from build123d import *

# Parameters (mm, degrees)
BOSS_EXTRUDE1_DEPTH     = 28
CUT_EXTRUDE1_DEPTH      = 19
CUT_EXTRUDE1_DEPTH_BACK = 52
SKETCH3_R               = 2.75
BOSS_EXTRUDE2_DEPTH     = 2
SKETCH5_R               = 2.25
CUT_EXTRUDE2_DEPTH      = 50
CUT_EXTRUDE3_DEPTH      = 2
MIRROR3_COPY_1_DEPTH    = 2
SKETCH7_R               = 7.5
CUT_EXTRUDE4_DEPTH      = 10
BOSS_EXTRUDE3_DEPTH     = 4
CHAMFER1_SIZE           = 4
SKETCH9_R               = 3.3
SKETCH9_R_2             = 2.75
BOSS_EXTRUDE4_DEPTH     = 1.5
CHAMFER2_SIZE           = 1.5
CHAMFER3_SIZE           = 1.5
SKETCH10_W              = 16
SKETCH10_H              = 4
BOSS_EXTRUDE5_DEPTH     = 28


with BuildPart() as part:
    # Sketch2 → Boss-Extrude1 (new body)
    with BuildSketch(Plane.XY):
        with BuildLine():
            ThreePointArc((-59.5, 14), (-56.717514421, 20.717514421), (-50, 23.5))
            Line((-50, 23.5), (-36, 23.5))
            Line((-36, 23.5), (-36, -19.5))
            Line((-36, -19.5), (-24, -19.5))
            Line((-24, -19.5), (-24, 23.5))
            Line((-24, 23.5), (50, 23.5))
            ThreePointArc((50, 23.5), (56.717514421, 20.717514421), (59.5, 14))
            Line((59.5, 14), (59.5, -14))
            ThreePointArc((59.5, -14), (56.717514421, -20.717514421), (50, -23.5))
            Line((50, -23.5), (-50, -23.5))
            ThreePointArc((-50, -23.5), (-56.717514421, -20.717514421), (-59.5, -14))
            Line((-59.5, -14), (-59.5, 14))
        make_face()
        with BuildLine():
            ThreePointArc((50, -19.5), (53.889087297, -17.889087297), (55.5, -14))
            Line((55.5, -14), (55.5, 14))
            ThreePointArc((55.5, 14), (53.889087297, 17.889087297), (50, 19.5))
            Line((50, 19.5), (-20, 19.5))
            Line((-20, 19.5), (-20, -19.5))
            Line((-20, -19.5), (50, -19.5))
        make_face(mode=Mode.SUBTRACT)
        with BuildLine():
            Line((-55.5, -14), (-55.5, 14))
            ThreePointArc((-55.5, 14), (-53.889087297, 17.889087297), (-50, 19.5))
            Line((-50, 19.5), (-40, 19.5))
            Line((-40, 19.5), (-40, -19.5))
            Line((-40, -19.5), (-50, -19.5))
            ThreePointArc((-50, -19.5), (-53.889087297, -17.889087297), (-55.5, -14))
        make_face(mode=Mode.SUBTRACT)
    extrude(amount=BOSS_EXTRUDE1_DEPTH)

    # Sketch3 → Cut-Extrude1 (cut, two sides: drawn at the far end of the back side and taken through both)
    with BuildSketch(Plane(origin=(-36, 0, 0), x_dir=(0, 0, -1), z_dir=(1, 0, 0)).offset(-CUT_EXTRUDE1_DEPTH_BACK)):
        with Locations(Location((-14, 1.5, 0), (0, 0, 180))):
            Circle(SKETCH3_R)
    extrude(amount=CUT_EXTRUDE1_DEPTH + CUT_EXTRUDE1_DEPTH_BACK, mode=Mode.SUBTRACT)

    # Sketch4 → Boss-Extrude2 (add)
    with BuildSketch(Plane.XY.offset(28)):
        with BuildLine():
            Line((50, 23.5), (-36, 23.5))
            Line((-36, 23.5), (-50, 23.5))
            ThreePointArc((-50, 23.5), (-56.717514421, 20.717514421), (-59.5, 14))
            Line((-59.5, 14), (-59.5, -14))
            ThreePointArc((-59.5, -14), (-56.717514421, -20.717514421), (-50, -23.5))
            Line((-50, -23.5), (50, -23.5))
            ThreePointArc((50, -23.5), (56.717514421, -20.717514421), (59.5, -14))
            Line((59.5, -14), (59.5, 14))
            ThreePointArc((59.5, 14), (56.717514421, 20.717514421), (50, 23.5))
        make_face()
    extrude(amount=BOSS_EXTRUDE2_DEPTH)

    # Sketch5 → Cut-Extrude2 (cut)
    with BuildSketch(Plane(origin=(0, 23.5, 0), x_dir=(1, 0, 0), z_dir=(0, 1, 0))):
        with Locations(Location((-50, -15, 0), (0, 0, 270))):
            Circle(SKETCH5_R)
    cut_extrude2 = extrude(amount=-CUT_EXTRUDE2_DEPTH, mode=Mode.SUBTRACT)

    # Sketch6 → Cut-Extrude3 (cut, symmetric)
    with BuildSketch(Plane(origin=(0, -19.5, 0), x_dir=(1, 0, 0), z_dir=(0, 1, 0))):
        Polygon((-50, -19.272391992), (-46.3, -17.136195996), (-46.3, -12.863804004), (-50, -10.727608008), (-53.7, -12.863804004), (-53.7, -17.136195996), align=None)
    cut_extrude3 = extrude(amount=CUT_EXTRUDE3_DEPTH, both=True, mode=Mode.SUBTRACT)

    # Mirror1: Cut-Extrude2 across plane
    add(cut_extrude2.mirror(Plane(origin=(0, 0, 0), x_dir=(0, 0, 1), z_dir=(1, 0, 0))), mode=Mode.SUBTRACT)

    # Mirror2: Cut-Extrude3 across plane
    add(cut_extrude3.mirror(Plane.ZX), mode=Mode.SUBTRACT)

    # Mirror3: Cut-Extrude3 across plane
    add(cut_extrude3.mirror(Plane(origin=(0, 0, 0), x_dir=(0, 0, 1), z_dir=(1, 0, 0))), mode=Mode.SUBTRACT)

    # Mirror3 copy 1 sketch → Mirror3 copy 1 (cut, symmetric)
    with BuildSketch(Plane(origin=(0, 19.5, 0), x_dir=(-1, 0, 0), z_dir=(0, -1, 0))):
        Polygon((-50, -19.272391992), (-46.3, -17.136195996), (-46.3, -12.863804004), (-50, -10.727608008), (-53.7, -12.863804004), (-53.7, -17.136195996), align=None)
    extrude(amount=MIRROR3_COPY_1_DEPTH, both=True, mode=Mode.SUBTRACT)

    # Sketch7 → Cut-Extrude4 (cut)
    with BuildSketch(Plane.ZY.offset(59.5)):
        with Locations((14, 1.5)):
            Circle(SKETCH7_R)
    extrude(amount=-CUT_EXTRUDE4_DEPTH, mode=Mode.SUBTRACT)

    # Sketch8 → Boss-Extrude3 (add)
    with BuildSketch(Plane(origin=(-20, 0, 0), x_dir=(0, 0, -1), z_dir=(1, 0, 0))):
        Polygon((-5.628421097, 1.5), (-9.814210548, 8.75), (-18.185789452, 8.75), (-22.371578903, 1.5), (-18.185789452, -5.75), (-9.814210548, -5.75), align=None)
        Polygon((-9.092522712, 1.5), (-11.546261356, 5.75), (-16.453738644, 5.75), (-18.907477288, 1.5), (-16.453738644, -2.75), (-11.546261356, -2.75), align=None, mode=Mode.SUBTRACT)
    extrude(amount=BOSS_EXTRUDE3_DEPTH)

    # Chamfer1
    chamfer1_edges = [part.edges().sort_by_distance(p)[0] for p in [
        (-20, 5.125, 7.721315823),
        (-20, 8.75, 14),
        (-20, 5.125, 20.278684177),
        (-20, -2.125, 20.278684177),
        (-20, -5.75, 14),
        (-20, -2.125, 7.721315823),
    ]]
    chamfer(chamfer1_edges, length=CHAMFER1_SIZE - 0.0001)  # a hair under: the kernel refuses the full size

    # Sketch9 → Boss-Extrude4 (add)
    with BuildSketch(Plane.ZY.offset(24)):
        with Locations((14, 1.5)):
            Circle(SKETCH9_R)
        with Locations((14, 1.5)):
            Circle(SKETCH9_R_2, mode=Mode.SUBTRACT)
    boss_extrude4 = extrude(amount=BOSS_EXTRUDE4_DEPTH)

    # Chamfer2
    chamfer2_edges = [part.edges().sort_by_distance(p)[0] for p in [
        (-24, 1.5, 10.7),
    ]]
    chamfer(chamfer2_edges, length=CHAMFER2_SIZE - 0.0001)  # a hair under: the kernel refuses the full size

    # Mirror6: Boss-Extrude4 across plane
    add(boss_extrude4.mirror(Plane(origin=(-30, 0, 0), x_dir=(0, 0, 1), z_dir=(1, 0, 0))))

    # Chamfer3
    chamfer3_edges = [part.edges().sort_by_distance(p)[0] for p in [
        (-36, 1.5, 10.7),
    ]]
    chamfer(chamfer3_edges, length=CHAMFER3_SIZE - 0.0001)  # a hair under: the kernel refuses the full size

    # Sketch10 → Boss-Extrude5 (add)
    with BuildSketch(Plane(origin=(0, 0, 0), x_dir=(-1, 0, 0), z_dir=(0, 0, -1))):
        with Locations((32, 21.5)):
            Rectangle(SKETCH10_W, SKETCH10_H)
    extrude(amount=-BOSS_EXTRUDE5_DEPTH)


solid = part.part
Work out the finished part from the listing and answer in its coordinate system (mm). A direction names the side the tool comes from. Coordinates: 2 decimals unless noted, no trailing zeros. Write each loop counter-clockwise with the first axis right and the second up, starting at its lowest first coordinate (ties: lowest second). Pieces come first, ordered by that corner, then holes. Notation, with made-up numbers: M 65,41 L 117,41 A13 ccw 117,45 Z; hole C -17.75,59 d11. An arc over 180 degrees is marked long. Answer as CSV lines item,"result". Start each with the question number.
Item 1: A tool of negligible diameter and unlimited length cuts with its end or side. For faces 1 (the face through (53.93, 17.85, 13.8)), 2 (the face through (47.77, -22.49, 14.71)), 3 (the face through (-46.3, 20, 15)), from which of +Z, -Z, +X, -X, +Y, -Y can it reach the whole face along a straight path? Write none if from no direction.
Item 2: Flat-ended cylindrical pins translate along their axes: P1, Ø1, axis at y = -20, z = 15.5, coming from the +X side; P2, Ø4, axis at x = -50, z = 15, coming from the -Y side; P3, Ø3.5, axis at x = -32.5, y = -1, coming from the -Z side. Find the tip coordinate at first contact, or state that the pin passes through.
Item 3: Section B-B on z = 15 is taken. Give the number of separate pieces and of enclosed holes in the cut face, and give its area (3 significant figures).
Item 4: Consider L1, parallel to X at y = -7.5, z = 23.5; L2, parallel to Z at x = 50, y = -22.05; L3, parallel to Z at x = 50, y = -21. Determine where each line is inside the solid, lowest interval first.
Item 5: Determine the mould class of faces 4 (the face through (59.5, 0, 15)), 5 (the face through (-57.528, -5.154, 17.461)) for opening direction Y: released by +Y, released by -Y, zero draft, split by the parting line, or undercut.
Item 6: Section A-A on x = 9.5 is taken. Write down the section's boundary in (y, z).
Checks:
1,face 1,"-Z"
1,face 2,"+Y, -Y"
1,face 3,"none"
2,P1,"stops at x = 57.75"
2,P2,"passes through"
2,P3,"stops at z = 28"
3,separate pieces,"5"
3,enclosed holes,"0"
3,area,"1,370 mm²"
4,L1,"x = -59.5 to -55.5, -40 to -36, -24 to -20, 55.5 to 59.5"
4,L2,"z = 0 to 12.75, 17.25 to 30"
4,L3,"z = 0 to 10.73, 19.27 to 30"
5,face 4,"zero draft"
5,face 5,"undercut"
6,outline,"M -23.5,0 L -19.5,0 L -19.5,28 L 19.5,28 L 19.5,0 L 23.5,0 L 23.5,30 L -23.5,30 Z"
